Input: part model. Units: mm. Frame: model coordinates. A direction names the side the tool comes from. Coordinates: 2 decimals unless noted, no trailing zeros. Order: outer loops, then holes, each group sorted by start corner. A loop starts at its lowest first (then second) coordinate and runs counter-clockwise, first axis right, second up.
from build123d import *

# Parameters (mm, degrees)
CROQUIS1_R              = 15
SALIENTE_EXTRUIR1_DEPTH = 50
CROQUIS2_R              = 4
SALIENTE_EXTRUIR2_DEPTH = 7.5
CORTAR_EXTRUIR2_START   = 8
CROQUIS3_R              = 4
CORTAR_EXTRUIR2_DEPTH   = 8
REDONDEO1_R             = 10
CORTAR_EXTRUIR3_DEPTH   = 15
CORTAR_EXTRUIR4_DEPTH   = 15
CROQUIS6_R              = 2.5
CORTAR_EXTRUIR5_DEPTH   = 15


with BuildPart() as part:
    # Croquis1 → Saliente-Extruir1 (new body)
    with BuildSketch(Plane(origin=(0, 0, 0), x_dir=(1, 0, 0), z_dir=(0, 1, 0))):
        with Locations(Location((0, 0, 0), (0, 0, 270))):
            Circle(CROQUIS1_R)
    extrude(amount=SALIENTE_EXTRUIR1_DEPTH)

    # Croquis2 → Saliente-Extruir2 (add, symmetric)
    with BuildSketch(Plane.XY):
        Circle(CROQUIS2_R)
    extrude(amount=SALIENTE_EXTRUIR2_DEPTH, both=True)

    # Croquis3 → Cortar-Extruir2 (cut)
    with BuildSketch(Plane.XY.offset(7.5).offset(CORTAR_EXTRUIR2_START)):
        Circle(CROQUIS3_R)
    cortar_extruir2 = extrude(amount=-CORTAR_EXTRUIR2_DEPTH, mode=Mode.SUBTRACT)

    # Simetría1: Cortar-Extruir2 across plane
    add(cortar_extruir2.mirror(Plane.XY), mode=Mode.SUBTRACT)

    # Redondeo1
    redondeo1_edges = [part.edges().sort_by_distance(p)[0] for p in [
        (0, 50, -15),
    ]]
    fillet(redondeo1_edges, radius=REDONDEO1_R)

    # Croquis4 → Cortar-Extruir3 (cut, symmetric)
    with BuildSketch(Plane.XY):
        Polygon((-15, 13.376474032), (-15, 0), (-4, 0), (-4, 3.567059742), align=None)
    extrude(amount=CORTAR_EXTRUIR3_DEPTH, both=True, mode=Mode.SUBTRACT)

    # Croquis5 → Cortar-Extruir4 (cut, symmetric)
    with BuildSketch(Plane.XY):
        with BuildLine():
            Line((0, 4), (-7.90720464, 4))
            Line((-7.90720464, 4), (-7.90720464, -4))
            Line((-7.90720464, -4), (0, -4))
            ThreePointArc((0, -4), (-4, 0), (0, 4))
        make_face()
    extrude(amount=CORTAR_EXTRUIR4_DEPTH, both=True, mode=Mode.SUBTRACT)

    # Croquis6 → Cortar-Extruir5 (cut)
    with BuildSketch(Plane.XY.offset(7.5)):
        Circle(CROQUIS6_R)
    extrude(amount=-CORTAR_EXTRUIR5_DEPTH, mode=Mode.SUBTRACT)


solid = part.part
Item 1: Ray query, probe 1 along X at (y, z) = (39.5, 4.5); probe 2 along Y at (x, z) = (-11.5, -4). Return the intervals inside material, ascending.
Response values:
probe 1: x = -14.31 to 14.31
probe 2: y = 10.26 to 46.96
Item 2: Access query for faces 1 (the face through (2, 2, 7.5)), 2 (the face through (-8.5, 7.58, 0.2)), 3 (the face through (8, 0, 0)), 4 (the face through (2, 2, -7.5)). Directions: +Z, -Z, +X, -X, +Y, -Y. A direction counts if a zero-diameter tool reaches every point of the face in a straight line with its end or side. Return the directions, or none.
Response values:
face 1: +Z, -X, -Y
face 2: +Z, -Z, -X, -Y
face 3: +Z, -Z, +X, -Y
face 4: -Z, -X, -Y
Item 3: Cut plane A-A on y = 19.5. Return loops of the section in (x, z).
Response values:
outline: circle Ø30 at (0, 0)
Item 4: Pin query (flat end, axial travel): pin 1 Ø5.5 at (x, z) = (8, -1) entering from -Y; pin 2 Ø3 at (y, z) = (24.5, -5) entering from +X; pin 3 Ø2 at (x, z) = (2.5, 9) entering from +Y. Return the tip coordinate at first contact, or that it passes through.
Response values:
pin 1: stops at y = 0
pin 2: stops at x = 14.59
pin 3: stops at y = 49.43
Item 5: Cut plane B-B on y = 7. Return loops of the section in (x, z), then the cut area to 3 significant figures.
Response values:
outline: (-7.85, -12.78) arc R15 ccw (long way) to (-7.85, 12.78) - close
area: 578 mm2
Item 6: Draft query along Y for faces 5 (the face through (0, 50, 0)), 6 (the face through (-0.54, -2.44, 0.11)), 7 (the face through (14.872, 19.72, -1.953)), 8 (the face through (2.859, 2.797, -11.302)). Return one class per face: pulls with the +Y half, pulls with the -Y half, needs draft (parallel to the pull), parting line crosses it, or undercut.
Response values:
face 5: pulls with the +Y half
face 6: undercut
face 7: needs draft
face 8: pulls with the -Y half
